Geometry: see drawing. Coordinates: mm, zero at the bounding-box minimum. Coordinates: 2 decimals unless noted, no trailing zeros. Order: outer loops, then holes, each group sorted by start corner. A loop starts at its lowest first (then second) coordinate and runs counter-clockwise, first axis right, second up. Notation, with made-up numbers: (-14, 1.5) -> (34, 1.5) arc R17 ccw to (34, 7.5) -> close; hole circle Ø6 at (80.5, 11.5). An arc over 180 degrees is marked (long way). Write each question's results on one line, items separated by ' | '.
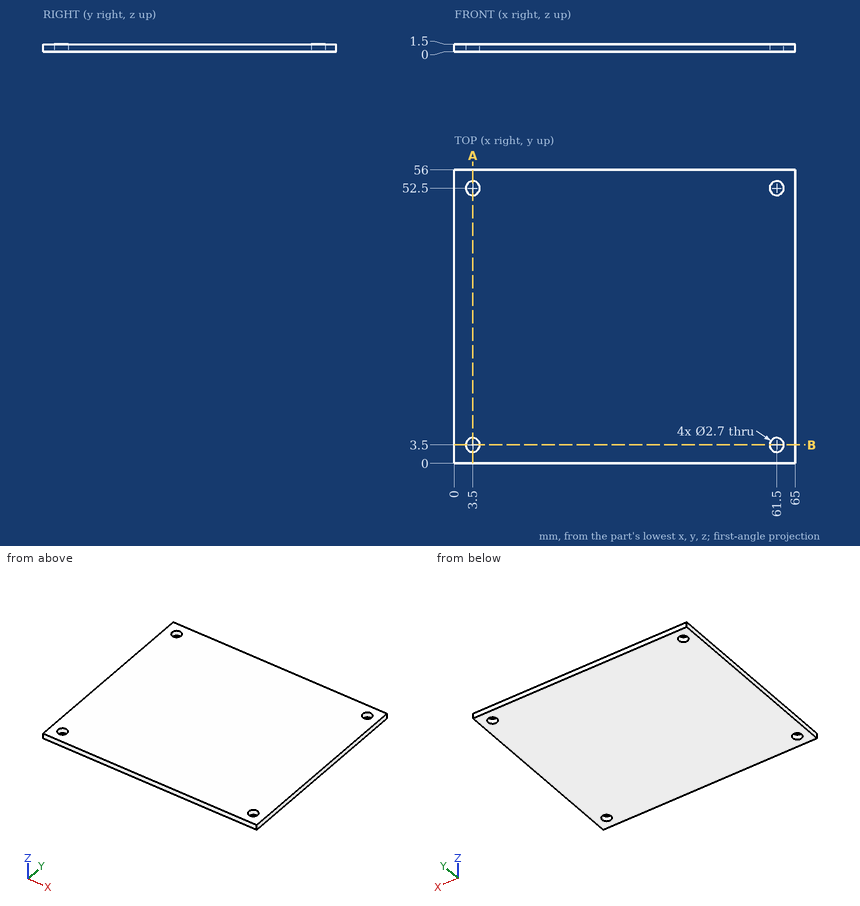
(1) Line query: line 1 along Y through (x, z) = (61.5, 0.3). Output: solid intervals per line, ascending. Write a range as from..to.
Return value:
line 1: 0..2.15, 4.85..51.15, 53.85..56
(2) Cut plane B-B, the plane y = 3.5. Return loops of the section in (x, z), plus the area to 3 significant figures.
Return value:
outline: (0, 0) -> (2.15, 0) -> (2.15, 1.5) -> (0, 1.5) -> close; (4.85, 0) -> (60.15, 0) -> (60.15, 1.5) -> (4.85, 1.5) -> close; (62.85, 0) -> (65, 0) -> (65, 1.5) -> (62.85, 1.5) -> close | area: 89.4 mm2
(3) Cut plane A-A, the plane x = 3.5. Return loops of the section in (y, z).
Return value:
outline: (0, 0) -> (2.15, 0) -> (2.15, 1.5) -> (0, 1.5) -> close; (4.85, 0) -> (51.15, 0) -> (51.15, 1.5) -> (4.85, 1.5) -> close; (53.85, 0) -> (56, 0) -> (56, 1.5) -> (53.85, 1.5) -> close
(4) Pin query (flat end, axial travel): P1, Ø10, axis at x = 25.5, y = 12, coming from the -Z side; P2, Ø1.6, axis at x = 61.5, y = 3.5, coming from the -Z side. Return the tip coordinate at first contact, or that it passes through.
Return value:
P1: z = 0 | P2: through
